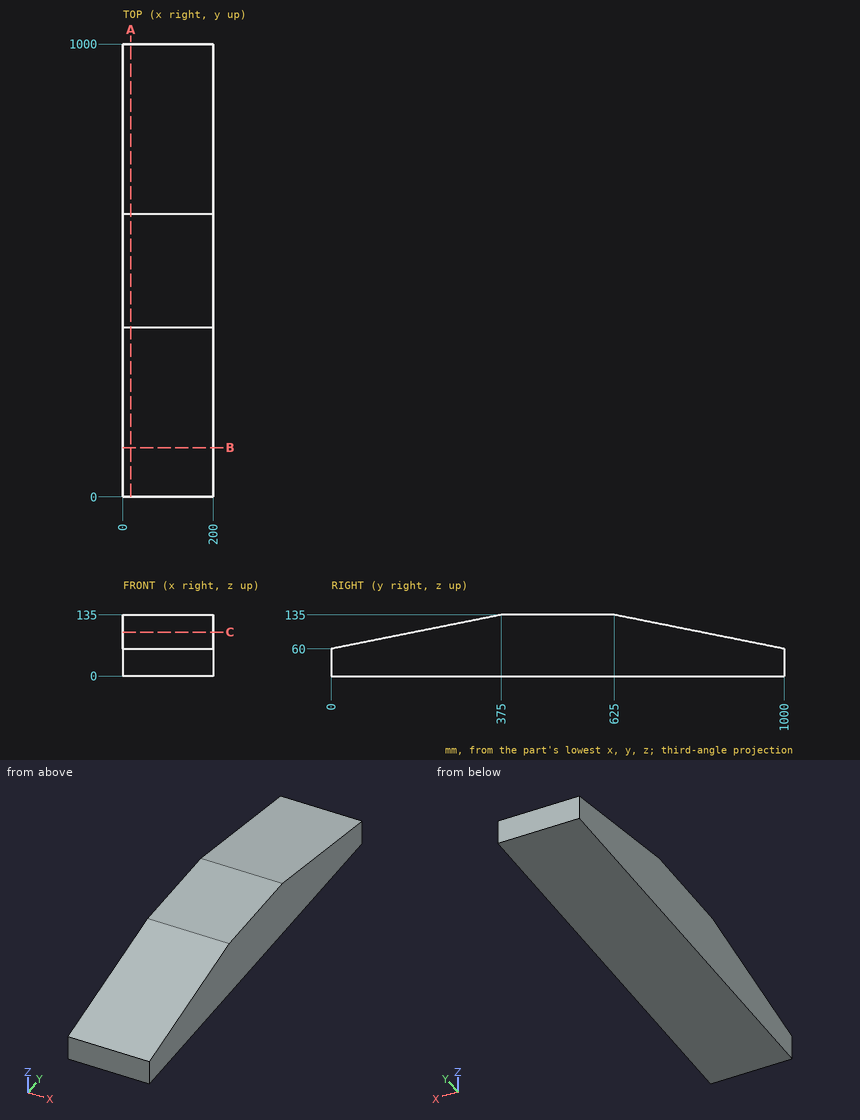
Answer from the drawing. Dimensions are ordinates in mm from the lowest x, y and z of the part. Coordinates: 2 decimals unless noted, no trailing zeros. Loops run counter-clockwise (first coordinate to the right, second up) from the corner with the lowest first, then second, coordinate; pieces in that order, holes last.
1) Section B-B (y = 109) is taken. Give the vertices of the cut face in (x, z), plus the area to 3 significant figures.
Results:
outline: (0, 0) - (200, 0) - (200, 81.8) - (0, 81.8) - close
area: 16,400 mm2
2) Section A-A (x = 18) is taken. Give the vertices of the cut face in (y, z).
Results:
outline: (0, 0) - (1000, 0) - (1000, 60) - (625, 135) - (375, 135) - (0, 60) - close
3) Section C-C (z = 97) is taken. Give the vertices of the cut face in (x, y).
Results:
outline: (0, 185) - (200, 185) - (200, 815) - (0, 815) - close
4) Consider probe 1 along Z at (x, y) = (86, 693.5); probe 2 along Z at (x, y) = (68.5, 726.5). Determine where each line is inside the solid, lowest interval first.
Results:
probe 1: z = 0 to 121.3
probe 2: z = 0 to 114.7
